Read the model definition and answer for the solid it produces. Units are mm, in the model's axes. Face numbers are marked on the shaded views. A direction names the side the tool comes from. Coordinates: 2 decimals unless noted, no trailing zeros. Loops run counter-clockwise (first coordinate to the right, second up) from the corner with the lowest first, then second, coordinate; pieces in that order, holes last. Notation, with made-up numbers: (75.5, 2) -> (110.5, 2) arc R23 cw to (110.5, 20) -> close; hole circle Ø4 at (32.5, 49.25). An arc over 180 degrees is marked (long way). Answer as a JSON object with one key per item and string values. Group by question number.
Q1. The part is cut by section C-C on z = 16.25. Write down the section's boundary in (x, y).
Q2. The part is cut by section A-A on y = 0. Write down the section's boundary in (x, z), and give its area (3 significant figures).
Q3. Straight lines are drawn through the part: line 1 along X through (y, z) = (0, 3.35); line 2 along Y through (x, z) = (0, 12); line 3 along Y through (x, z) = (-15.5, 10.75). For each, find the intervals that lie inside material, in ascending order. Write a range as [from, to].
Q4. The part is cut by section D-D on y = 10.5. Write down the section's boundary in (x, z).
Q5. The part is cut by section B-B on x = 13.5. Write down the section's boundary in (y, z), and give its area (3 significant figures).
Q6. Each of these flat-tipped pins is pushed along its axis until it touches: P1, Ø1, axis at x = 10.5, z = 9.5, coming from the -Y side; P2, Ø3, axis at y = 5, z = 16, coming from the +X side; P3, Ø1.7, axis at x = 30.9, y = 0, coming from the -Z side. Where does it stop, or does it pass through?
Q7. For the marked faces 4 and 5, determine the directions among +Z, -Z, +X, -X, +Y, -Y from which every point of the face is accessible in a straight line to the end or side of a thin tool.
Q8. Determine the mould class of the marked faces 1, 2 and 3 for opening direction X: released by +X, released by -X, zero draft, split by the parting line, or undercut.
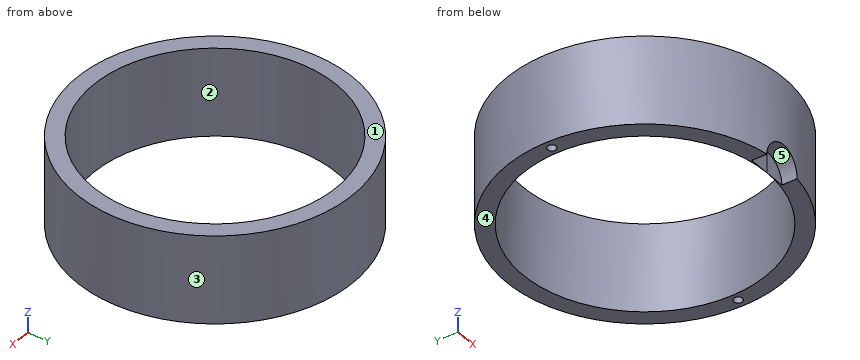
from build123d import *

# Parameters (mm, degrees)
CYLINDER_R     = 5
CYLINDER_DEPTH = 10
TUBE_R         = 33
TUBE_R_2       = 29
TUBE_DEPTH     = 21
SKETCH001_R    = 1.032289
POCKET_DEPTH   = 5


with BuildPart() as cylinder:
    # Cylinder → Cylinder (new body)
    with BuildSketch(Plane.XZ.offset(29)):
        Circle(CYLINDER_R)
    extrude(amount=CYLINDER_DEPTH)


with BuildPart() as body004:
    # Tube → Tube (new body)
    with BuildSketch(Plane.XY):
        Circle(TUBE_R)
        Circle(TUBE_R_2, mode=Mode.SUBTRACT)
    extrude(amount=TUBE_DEPTH)

    # Cut: cut Cylinder
    add(cylinder.part, mode=Mode.SUBTRACT)

    # Sketch001 (on DatumPlane) → Pocket (cut)
    with BuildSketch(Plane(origin=(0, 0, 0), x_dir=(1, 0, 0), z_dir=(0, 0, -1))):
        with Locations((-30.899429, 0)):
            Circle(SKETCH001_R)
    pocket = extrude(amount=-POCKET_DEPTH, mode=Mode.SUBTRACT)

    # Mirrored: Pocket across Sketch001 V_Axis
    add(pocket.mirror(Plane(origin=(0, 0, 0), x_dir=(0, 0, -1), z_dir=(1, 0, 0))), mode=Mode.SUBTRACT)


solid = body004.part
Final values:
{
 "1": {"outline": "circle Ø66 at (0, 0); hole circle Ø58 at (0, 0)"},
 "2": {"outline": "(-33, 0) -> (-31.93, 0) -> (-31.93, 5) -> (-29.87, 5) -> (-29.87, 0) -> (-29, 0) -> (-29, 21) -> (-33, 21) -> close; (29, 0) -> (29.87, 0) -> (29.87, 5) -> (31.93, 5) -> (31.93, 0) -> (33, 0) -> (33, 21) -> (29, 21) -> close", "area": "147 mm2"},
 "3": {"line 1": "x = [-33, -31.93], [-29.87, -29], [29, 29.87], [31.93, 33]", "line 2": "y = [-33, -29], [29, 33]", "line 3": "y = [-29.13, -24.51], [24.51, 29.13]"},
 "4": {"outline": "(-31.28, 0) -> (-27.03, 0) -> (-27.03, 21) -> (-31.28, 21) -> close; (27.03, 0) -> (31.28, 0) -> (31.28, 21) -> (27.03, 21) -> close"},
 "5": {"outline": "(-30.11, 0) -> (-25.67, 0) -> (-25.67, 21) -> (-30.11, 21) -> close; (25.67, 0) -> (30.11, 0) -> (30.11, 21) -> (25.67, 21) -> close", "area": "187 mm2"},
 "6": {"P1": "stops at y = -31.45", "P2": "stops at x = 32.81", "P3": "stops at z = 5"},
 "7": {"face 4": "-Z, +X, -X, +Y, -Y", "face 5": "-Z, -Y"},
 "8": {"face 1": "zero draft", "face 2": "undercut", "face 3": "split by the parting line"}
}
